Part model, mm, in its own coordinate system. Face numbers are marked on the shaded views. A direction names the side the tool comes from. Round coordinates to 2 decimals unless told otherwise and drop trailing zeros. Write each loop counter-clockwise with the first axis right and the second up, starting at its lowest first coordinate (ties: lowest second). Pieces come first, ordered by that corner, then holes. Notation, with made-up numbers: M 79,42 L 138,42 A7 cw 138,49 Z; hole C 48.25,-19 d10. An arc over 180 degrees is marked long. Use a Markdown table: item, result. Add a question column.
1) Slice it at B-B on x = -24. Write the cut outline in (y, z), plus the area to 3 significant figures.
2) Which spindle directions (+Z, -Z, +X, -X, +Y, -Y) get a long thin tool onto all of the face, cutting with end or side? Do the marked faces 1 and 2. Say none if no direction does.
3) Drop flat-ended pins along their axis: P1, Ø4, axis at x = 9, y = 6, coming from the +Z side; P2, Ø5.5, axis at x = 21.5, y = 30, coming from the -Z side; P3, Ø0.6, axis at x = -13.5, y = 13, coming from the +Z side. Give the stop position or say it passes through.
4) Wall check: probe 1 along Y at (x, z) = (24, 4.75); probe 2 along X at (y, z) = (17, -10.75); probe 3 along X at (y, z) = (12, -5.25). Give the ranges that are in metal, low to high.
5) Slice it at A-A on z = 6.25. Write the cut outline in (x, y), plus the area to 3 significant figures.
6) Slice it at C-C on y = 29.5. Write the cut outline in (x, z), plus the area to 3 significant figures.
7) Two-plate mould, pull along X, no slides. Class the marked faces 3, 4 and 5: released by +X, released by -X, zero draft, split by the parting line, or undercut.
8) Slice it at D-D on z = -10. Write the cut outline in (x, y).
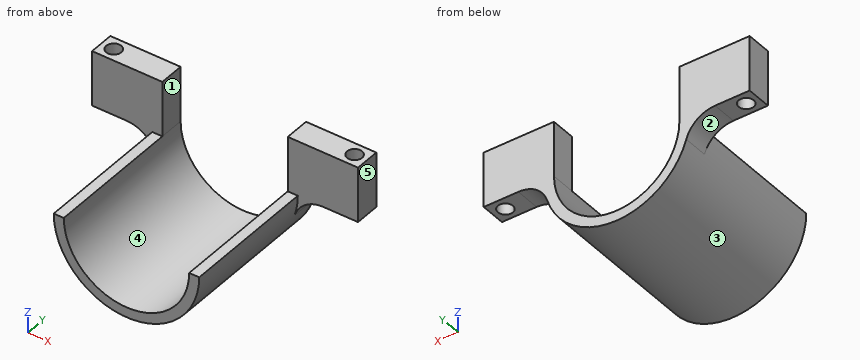
```python
from build123d import *

# Parameters (mm, degrees)
BOSS_EXTRUDE1_DEPTH = 32
BOSS_EXTRUDE2_DEPTH = 11
SKETCH3_R           = 1.5
CUT_EXTRUDE1_DEPTH  = 45.005681451
FILLET1_R           = 6


with BuildPart() as part:
    # Sketch1 → Boss-Extrude1 (new body)
    with BuildSketch(Plane(origin=(0, 0, 0), x_dir=(1, 0, 0), z_dir=(0, 1, 0))):
        with BuildLine():
            Line((-14.5, 0), (-12.5, 0))
            ThreePointArc((-12.5, 0), (0, 12.5), (12.5, 0))
            Line((12.5, 0), (14.5, 0))
            ThreePointArc((14.5, 0), (0, 14.5), (-14.5, 0))
        make_face()
    extrude(amount=BOSS_EXTRUDE1_DEPTH)

    # Sketch2 → Boss-Extrude2 (add)
    with BuildSketch(Plane.XY):
        Polygon((-14.5, 32), (-12.5, 32), (-12.5, 27), (-14.5, 27), (-26.5, 27), (-26.5, 32), align=None)
        Polygon((12.5, 32), (12.5, 27), (14.5, 27), (26.5, 27), (26.5, 32), (14.5, 32), align=None)
    extrude(amount=BOSS_EXTRUDE2_DEPTH)

    # Sketch3 → Cut-Extrude1 (cut, through all)
    with BuildSketch(Plane(origin=(0, 0, 0), x_dir=(-1, 0, 0), z_dir=(0, 0, -1))):
        with Locations((24, 29.5)):
            Circle(SKETCH3_R)
        with Locations(Location((-24, 29.5, 0), (0, 0, 180))):
            Circle(SKETCH3_R)
    extrude(amount=-CUT_EXTRUDE1_DEPTH, mode=Mode.SUBTRACT)

    # Fillet1
    fillet1_edges = [part.edges().sort_by_distance(p)[0] for p in [
        (-14.5, 29.5, 0),
        (14.5, 29.5, 0),
    ]]
    fillet(fillet1_edges, radius=FILLET1_R)


solid = part.part
```
Entries:
| question | item | result |
|---|---|---|
| 1 | outline | M 27,0 L 28,0 L 28,11 L 27,11 Z; M 31,0 L 32,0 L 32,11 L 31,11 Z |
| 1 | area | 22.0 mm^2 |
| 2 | face 1 | +Z, +Y, -Y |
| 2 | face 2 | -Z, -X, +Y, -Y |
| 3 | P1 | stops at z = -5.94 |
| 3 | P2 | stops at z = -0.06 |
| 3 | P3 | stops at z = 0 |
| 4 | probe 1 | y = 27 to 28, 31 to 32 |
| 4 | probe 2 | x = -9.73 to -6.38, 6.38 to 9.73 |
| 4 | probe 3 | x = -13.52 to -11.34, 11.34 to 13.52 |
| 5 | outline | M -26.5,27 L -12.5,27 L -12.5,32 L -26.5,32 Z; M 12.5,27 L 26.5,27 L 26.5,32 L 12.5,32 Z; hole C -24,29.5 d3; hole C 24,29.5 d3 |
| 5 | area | 126 mm^2 |
| 6 | outline | M -26.5,0 L -25.5,0 L -25.5,11 L -26.5,11 Z; M -22.5,0 L -19.6,0 A6 cw -13.87,-4.24 A14.5 ccw 13.87,-4.24 A6 cw 19.6,0 L 22.5,0 L 22.5,11 L 12.5,11 L 12.5,0 A12.5 cw -12.5,0 L -12.5,11 L -22.5,11 Z; M 25.5,0 L 26.5,0 L 26.5,11 L 25.5,11 Z |
| 6 | area | 336 mm^2 |
| 7 | face 3 | split by the parting line |
| 7 | face 4 | undercut |
| 7 | face 5 | released by +X |
| 8 | outline | M -10.5,0 L -7.5,0 L -7.5,32 L -10.5,32 Z; M 7.5,0 L 10.5,0 L 10.5,32 L 7.5,32 Z |
